Build history of the part. All positions in model axes, mm. A direction names the side the tool comes from. Coordinates: 2 decimals unless noted, no trailing zeros. Loops run counter-clockwise (first coordinate to the right, second up) from the corner with the lowest first, then second, coordinate; pieces in that order, holes last.
(1) Two-plate mould, pull along X, no slides. Class faces 1 (the face through (-16, 0, 1)), 2 (the face through (10, 17.5, 1)), 3 (the face through (0, 10, 1)): pulls with the +X half, pulls with the -X half, needs draft (parallel to the pull), parting line crosses it, or undercut.
(2) Flat gauge pins, fed straight in: P1, Ø0.6, axis at y = -16.5, z = 1.5, coming from the +X side; P2, Ø1, axis at x = 0.5, z = 1.5, coming from the -Y side; P3, Ø0.9, axis at y = 0.5, z = 2, coming from the +X side. Where does each tip first touch, or does it go through?
(3) Slice it at C-C (z = 1.85). Give the number of separate pieces and of enclosed holes in the cut face, and give its area (3 significant figures).
(4) Slice it at D-D (y = -2). Give the cut face in (x, z).
(5) Wall check: L1, parallel to Y at x = 0, z = 1.7; L2, parallel to X at y = 1, z = 0.6. Give the ranges that are in metal, low to high.
(6) Slice it at A-A (y = 12). Give the cut face in (x, z).
(7) Slice it at B-B (x = 0). Give the cut face in (y, z).
(8) Tool access for faces 4 (the face through (0, 16, 1)), 5 (the face through (-16.07, 16, 1.48)), 6 (the face through (2, 6, 2)), 7 (the face through (16, 0, 1)): list every direction of +Z, -Z, +X, -X, +Y, -Y with a clear straight run to the whole face (end or side of a thin tool).
Autodesk Inventor part; units mm, degrees
ref_plane "YZ Plane" through (0, 0, 0) normal (1, 0, 0) x (0, 1, 0)
ref_plane "XZ Plane" through (0, 0, 0) normal (0, 1, 0) x (-1, 0, 0)
ref_plane "XY Plane" through (0, 0, 0) normal (0, 0, 1) x (1, 0, 0)
sketch "Sketch1" plane through (0, 0, 0) normal (0, 0, 1) x (1, 0, 0)
  circle A0 centre (0, 12) radius 2
  line L0 (-17, -6) -> (-16.5, -6)
  line L1 (-16, -5.5) -> (-16, 5.5)
  line L2 (-16.5, 6) -> (-17, 6)
  line L3 (-17.5, 12.5) -> (-17.5, 6.5)
  line L4 (-17.5, -6.5) -> (-17.5, -12.5)
  arc A1 (-16.5, -6) -> (-16, -5.5) centre (-16.5, -5.5) ccw
  arc A2 (-16, 5.5) -> (-16.5, 6) centre (-16.5, 5.5) ccw
  arc A3 (-17.5, 6.5) -> (-17, 6) centre (-17, 6.5) ccw
  arc A4 (-17, -6) -> (-17.5, -6.5) centre (-17, -6.5) ccw
  line L5 (6, -17) -> (6, -16.5)
  line L6 (5.5, -16) -> (-5.5, -16)
  line L7 (-6, -16.5) -> (-6, -17)
  arc A5 (6, -16.5) -> (5.5, -16) centre (5.5, -16.5) ccw
  arc A6 (-5.5, -16) -> (-6, -16.5) centre (-5.5, -16.5) ccw
  arc A7 (-6.5, -17.5) -> (-6, -17) centre (-6.5, -17) ccw
  arc A8 (6, -17) -> (6.5, -17.5) centre (6.5, -17) ccw
  line L8 (17, 6) -> (16.5, 6)
  line L9 (16, 5.5) -> (16, -5.5)
  line L10 (16.5, -6) -> (17, -6)
  arc A9 (16.5, 6) -> (16, 5.5) centre (16.5, 5.5) ccw
  arc A10 (16, -5.5) -> (16.5, -6) centre (16.5, -5.5) ccw
  arc A11 (17.5, -6.5) -> (17, -6) centre (17, -6.5) ccw
  arc A12 (17, 6) -> (17.5, 6.5) centre (17, 6.5) ccw
  line L11 (-6, 17) -> (-6, 16.5)
  line L12 (-5.5, 16) -> (5.5, 16)
  line L13 (6, 16.5) -> (6, 17)
  arc A13 (-6, 16.5) -> (-5.5, 16) centre (-5.5, 16.5) ccw
  arc A14 (5.5, 16) -> (6, 16.5) centre (5.5, 16.5) ccw
  arc A15 (6.5, 17.5) -> (6, 17) centre (6.5, 17) ccw
  arc A16 (-6, 17) -> (-6.5, 17.5) centre (-6.5, 17) ccw
  line L14 (12.5, 17.5) -> (6.5, 17.5)
  line L15 (-6.5, 17.5) -> (-12.5, 17.5)
  line L16 (17.5, -12.5) -> (17.5, -6.5)
  line L17 (17.5, 6.5) -> (17.5, 12.5)
  line L18 (-12.5, -17.5) -> (-6.5, -17.5)
  line L19 (6.5, -17.5) -> (12.5, -17.5)
  arc A17 (-17.5, -12.5) -> (-12.5, -17.5) centre (-12.5, -12.5) ccw
  arc A18 (-12.5, 17.5) -> (-17.5, 12.5) centre (-12.5, 12.5) ccw
  arc A19 (17.5, 12.5) -> (12.5, 17.5) centre (12.5, 12.5) ccw
  arc A20 (12.5, -17.5) -> (17.5, -12.5) centre (12.5, -12.5) ccw
  point P0 (0, 0)
  point P1 (16, 0)
  point P2 (-16, 6)
  point P3 (-16, -6)
  point P4 (-16, 0)
  point P5 (-6, -16)
  point P6 (6, -16)
  point P7 (0, -16)
  point P8 (16, -6)
  point P9 (16, 6)
  point P10 (6, 16)
  point P11 (-6, 16)
  point P12 (0, 16)
  dimension "d6" = 4
  dimension "d44" = 12
  dimension "d45" = 0.5
  dimension "d48" = 360
  dimension "d50" = 5
  dimension "d64" = 12
  dimension "d65" = 16
  dimension "d66" = 35
extrude "Extrusion6" add sketch "Sketch1" along normal blind 3
sketch "Sketch4" plane through (0, 0, 3) normal (0, 0, 1) x (1, 0, 0)
  line L0 (-1, 7) -> (1, 7)
  line L1 (2, 6) -> (2, 6)
  line L2 (1, 5) -> (-1, 5)
  line L3 (-2, 6) -> (-2, 6)
  arc A0 (-1, 7) -> (-2, 6) centre (-1, 6) ccw
  arc A1 (2, 6) -> (1, 7) centre (1, 6) ccw
  arc A2 (1, 5) -> (2, 6) centre (1, 6) ccw
  arc A3 (-2, 6) -> (-1, 5) centre (-1, 6) ccw
  point P0 (0, 0)
  point P1 (-2, 7)
  point P2 (2, 5)
  point P3 (-2, 5)
  point P4 (0, 5)
  dimension "d76" = 2
  dimension "d77" = 4
  dimension "d78" = 5
  dimension "d79" = 1
extrude "Extrusion8" cut sketch "Sketch4" against normal through all
properties part number "020914 Aft Outer Endcap" material "Polycarbonate, Clear"
Response values:
1. face 1: pulls with the -X half
1. face 2: needs draft
1. face 3: undercut
2. P1: stops at x = 15.86
2. P2: stops at y = -16
2. P3: stops at x = 16
3. separate pieces: 1
3. enclosed holes: 2
3. area: 1,110 mm2
4. outline: (-16, 0) - (16, 0) - (16, 3) - (-16, 3) - close
5. L1: y = -16 to 5, 7 to 10, 14 to 16
5. L2: x = -16 to 16
6. outline: (-17.5, 0) - (-2, 0) - (-2, 3) - (-17.5, 3) - close; (2, 0) - (17.5, 0) - (17.5, 3) - (2, 3) - close
7. outline: (-16, 0) - (5, 0) - (5, 3) - (-16, 3) - close; (7, 0) - (10, 0) - (10, 3) - (7, 3) - close; (14, 0) - (16, 0) - (16, 3) - (14, 3) - close
8. face 4: +Z, -Z, +Y
8. face 5: +Z, -Z, -X, +Y
8. face 6: +Z, -Z
8. face 7: +Z, -Z, +X
